```python
from build123d import *

# Parameters (mm, degrees)
SKETCH1_R                      = 6.35
SKETCH1_R_2                    = 1.35255
EXTRUDE1_DEPTH                 = 19.812
EXTRUDE1_DEPTH_BACK            = 19.812
CUT_EXTRUDE1_REACH             = 8.35
SKETCH3_R                      = 1.89865
CUT_EXTRUDE1_DIRECTION_2_REACH = 8.35


with BuildPart() as part:
    # Sketch1 → Extrude1 (new body, two sides)
    with BuildSketch(Plane(origin=(0, 0, 0), x_dir=(1, 0, 0), z_dir=(0, 1, 0))) as extrude1_sk:
        Circle(SKETCH1_R)
        Circle(SKETCH1_R_2, mode=Mode.SUBTRACT)
    extrude(amount=EXTRUDE1_DEPTH)
    extrude(extrude1_sk.sketch, amount=-EXTRUDE1_DEPTH_BACK)

    # Sketch3 → Cut-Extrude1 (cut, up to next)
    with BuildSketch(Plane(origin=(0, 0, 0), x_dir=(0, 0, -1), z_dir=(1, 0, 0)), mode=Mode.PRIVATE) as cut_extrude1_sk1:
        Circle(SKETCH3_R)
    cut_extrude1_tool1 = extrude(cut_extrude1_sk1.sketch, amount=-CUT_EXTRUDE1_REACH, mode=Mode.PRIVATE) & part.part
    add(cut_extrude1_tool1.solids().sort_by_distance((0, 0, 0))[0], mode=Mode.SUBTRACT)

    # Sketch3 → Cut-Extrude1 direction 2 (cut, up to next)
    with BuildSketch(Plane(origin=(0, 0, 0), x_dir=(0, 0, -1), z_dir=(1, 0, 0)), mode=Mode.PRIVATE) as cut_extrude1_direction_2_sk1:
        Circle(SKETCH3_R)
    cut_extrude1_direction_2_tool1 = extrude(cut_extrude1_direction_2_sk1.sketch, amount=CUT_EXTRUDE1_DIRECTION_2_REACH, mode=Mode.PRIVATE) & part.part
    add(cut_extrude1_direction_2_tool1.solids().sort_by_distance((0, 0, 0))[0], mode=Mode.SUBTRACT)


solid = part.part
```
Geometry check sheet. Reference: the model listing, model coordinates, mm. Give positions to 0.01 mm unless a question says otherwise; leave off trailing zeros. Write each loop counter-clockwise with the first axis right and the second up, starting at its lowest first coordinate (ties: lowest second). Pieces come first, ordered by that corner, then holes.
1) Section check C-C, the plane y = -12.5. Record the boundary of the cut face in (x, z), and give its area (3 significant figures).
2) Gauge pin test, flat ends, axial feed: pin 1 (4 mm diameter, centred on y = 6, z = 2.5, fed in from -X); pin 2 (1 mm diameter, centred on y = 5.5, z = -2.5, fed in from +X); pin 3 (3 mm diameter, centred on y = -2, z = 5, fed in from +X). Record the tip position at first contact, or that the pin passes through.
3) Section check D-D, the plane y = 0. Record the boundary of the cut face in (x, z), and give its area (3 significant figures).
4) Material ranges on L1, parallel to X at y = -7.5, z = 0; L2, parallel to X at y = 17.5, z = 0.25, recorded low to high.
5) Release check for a two-part mould opening along Z. For faces 1 (the cylindrical face through (5.866, 0.277, 2.432)), 2 (the flat face through (0, -19.812, -2)), 3 (the cylindrical face through (1.29, -10.44, -0.41)) record: pulls with the +Z half, pulls with the -Z half, needs draft (parallel to the pull), parting line crosses it, or undercut.
6) Section check A-A, the plane z = 0. Record the boundary of the cut face in (x, y), and give its area (3 significant figures).
7) Section check B-B, the plane x = 2.75. Record the boundary of the cut face in (y, z).
Computed:
1. outline: circle Ø12.7 at (0, 0); hole circle Ø2.71 at (0, 0)
1. area: 121 mm2
2. pin 1: stops at x = -6.33
2. pin 2: stops at x = 6.03
2. pin 3: stops at x = 5.3
3. outline: (-6.06, -1.9) arc R6.35 ccw to (6.06, -1.9) - close; (-6.06, 1.9) - (6.06, 1.9) arc R6.35 ccw to start
3. area: 79.2 mm2
4. L1: x = -6.35 to -1.35, 1.35 to 6.35
4. L2: x = -6.35 to -1.33, 1.33 to 6.35
5. face 1: parting line crosses it
5. face 2: needs draft
5. face 3: undercut
6. outline: (-6.35, -19.81) - (-1.35, -19.81) - (-1.35, -1.9) - (-6.35, -1.9) - close; (-6.35, 1.9) - (-1.35, 1.9) - (-1.35, 19.81) - (-6.35, 19.81) - close; (1.35, -19.81) - (6.35, -19.81) - (6.35, -1.9) - (1.35, -1.9) - close; (1.35, 1.9) - (6.35, 1.9) - (6.35, 19.81) - (1.35, 19.81) - close
6. area: 358 mm2
7. outline: (-19.81, -5.72) - (19.81, -5.72) - (19.81, 5.72) - (-19.81, 5.72) - close; hole circle Ø3.8 at (0, 0)
